Answer from the drawing. Dimensions are ordinates in mm from the lowest x, y and z of the part. A direction names the side the tool comes from. Round coordinates to 2 decimals unless told otherwise and drop trailing zeros. Loops run counter-clockwise (first coordinate to the right, second up) from the corner with the lowest first, then second, coordinate; pieces in that order, holes last. Notation, with made-up numbers: (-36.75, 1) - (17.25, 1) arc R27 cw to (17.25, 17) - close; hole circle Ø8 at (57, 73). An arc over 180 degrees is marked (long way). Return JSON: item names as keys, results as strings.
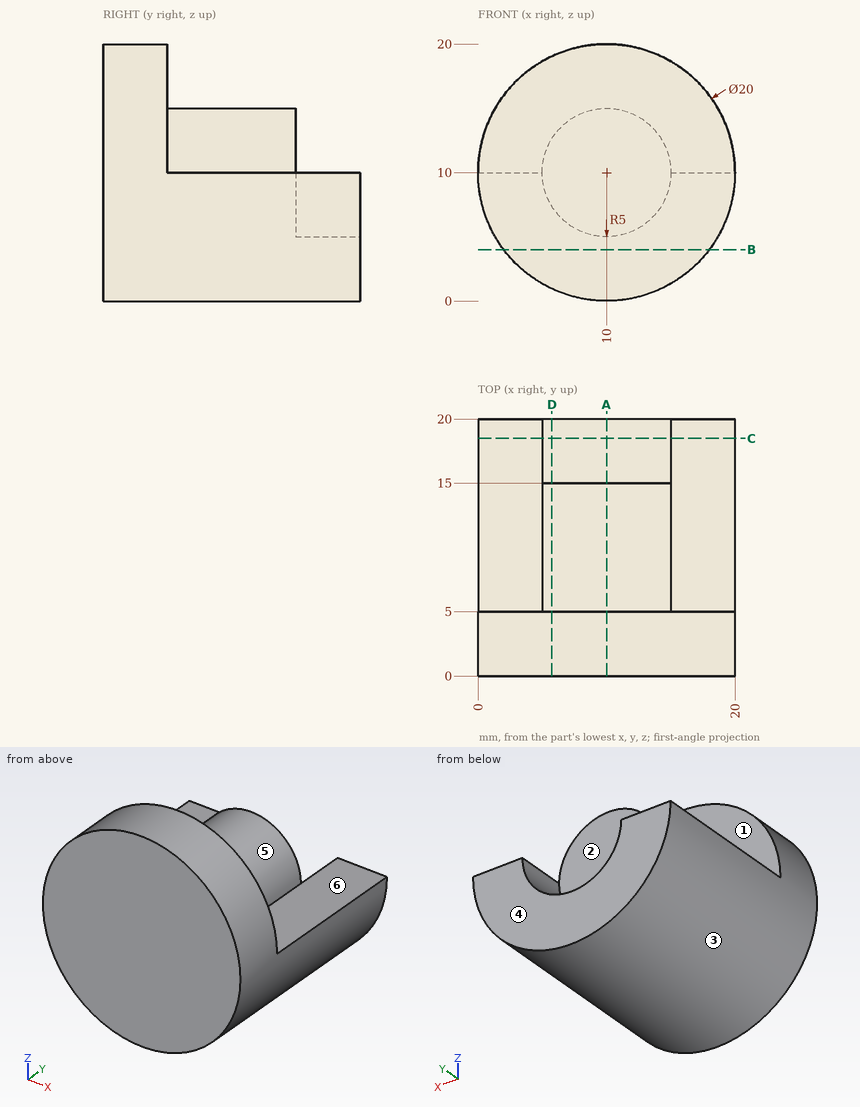
1) Section C-C (y = 18.5) is taken. Give the vertices of the cut face in (x, z), and give its area (3 significant figures).
Verdict:
{"outline": "(0, 10) arc R10 ccw to (20, 10) - (15, 10) arc R5 cw to (5, 10) - close", "area": "118 mm2"}
2) A tool of negligible diameter and unlimited length cuts with its end or side. For the marked faces 4, 5 and 6, from which of +Z, -Z, +X, -X, +Y, -Y can it reach the whole face along a straight path? Write none if from no direction.
Verdict:
{"face 4": "+Z, -Z, +X, -X, +Y", "face 5": "+Z, +Y", "face 6": "+Z, +X, +Y"}
3) Section B-B (z = 4) is taken. Give the vertices of the cut face in (x, y), and give its area (3 significant figures).
Verdict:
{"outline": "(2, 0) - (18, 0) - (18, 20) - (2, 20) - close", "area": "320 mm2"}
4) Find the intervals of material crossed by L1, parallel to Y at x = 7.75, z = 13.25; L2, parallel to Z at x = 10, y = 2.25; L3, parallel to X at y = 6, z = 10.25, in increasing order.
Verdict:
{"L1": "y = 0 to 15", "L2": "z = 0 to 20", "L3": "x = 5.01 to 14.99"}
5) Section D-D (x = 5.75) is taken. Give the vertices of the cut face in (y, z), and give its area (3 significant figures).
Verdict:
{"outline": "(0, 0.95) - (20, 0.95) - (20, 7.37) - (15, 7.37) - (15, 12.63) - (5, 12.63) - (5, 19.05) - (0, 19.05) - close", "area": "239 mm2"}
6) Flat-ended cylindrical pins translate along their axes: pin 1 (4 mm diameter, centred on x = 13, y = 7.5, fed in from -Z); pin 2 (3 mm diameter, centred on y = 5.5, z = 2.5, fed in from -X); pin 3 (5.5 mm diameter, centred on x = 18.5, y = 14.5, fed in from +Z). Find the tip coordinate at first contact, or state that the pin passes through.
Verdict:
{"pin 1": "stops at z = 0.05", "pin 2": "stops at x = 2", "pin 3": "stops at z = 10"}
7) Determine the mould class of the marked faces 1, 2 and 3 for opening direction X: pulls with the +X half, pulls with the -X half, needs draft (parallel to the pull), parting line crosses it, or undercut.
Verdict:
{"face 1": "needs draft", "face 2": "undercut", "face 3": "parting line crosses it"}
8) Section A-A (x = 10) is taken. Give the vertices of the cut face in (y, z), and give its area (3 significant figures).
Verdict:
{"outline": "(0, 0) - (20, 0) - (20, 5) - (15, 5) - (15, 15) - (5, 15) - (5, 20) - (0, 20) - close", "area": "275 mm2"}
